```python
from build123d import *

# Parameters (mm, degrees)
SKETCH_1_R = 1


with BuildPart() as part:
    # По траектории1: sweep along a curve in space
    with BuildLine() as sweep_1_path:
        Line((0, 0, 0), (10, 0, 0))
        ThreePointArc((10, 0, 0), (12.121320344, 0, -0.878679656), (13, 0, -3))
        Line((13, 0, -3), (13, 0, -23))
        ThreePointArc((13, 0, -23), (12.121320344, 0, -25.121320344), (10, 0, -26))
        Line((10, 0, -26), (-0.116555464, 0, -26))
    # Эскиз1 → По траектории1 (sweep)
    with BuildSketch(Plane(origin=(0, 0, 0), x_dir=(0, 0, -1), z_dir=(1, 0, 0))):
        Circle(SKETCH_1_R)
    sweep(path=sweep_1_path.line)


solid = part.part
```
The listing builds one solid part. Answer for the finished solid, in the listing's coordinates (mm). A direction names the side the tool comes from. Coordinates: 2 decimals unless noted, no trailing zeros. Loops run counter-clockwise (first coordinate to the right, second up) from the corner with the lowest first, then second, coordinate; pieces in that order, holes last. Notation, with made-up numbers: (-27, 84.25) - (8, 84.25) arc R25 cw to (8, 107.25) - close; hole circle Ø9 at (20.5, 33). An arc over 180 degrees is marked (long way). Use a Markdown table: item, result. Add a question column.
1) Find the intervals of material crossed by line 1 (Z direction, x = 5.25, y = 0.15); line 2 (Z direction, x = 8.75, y = -0.45); line 3 (X direction, y = 0.6, z = -7.5), in increasing order.
2) The mould has two halves that part along Z. Classify faces 3 (the cylindrical face through (5, -1, 0)), 4 (the cylindrical face through (12, 0, -13)), 5 (the flat face through (-0.117, 0, -26)): released by +Z, released by -Z, zero draft, split by the parting line, or undercut.
3) The part is cut by section A-A, the plane y = 0.6. Give the vertices of the cut face in (x, z), and give its area (3 significant figures).
4) Given pin 1 (1 mm diameter, centred on y = 0, z = -0.5, fed in from -X), flat-ended and moving along its own axis, determine where the tip first touches the part or whether it passes through.
5) The part is cut by section C-C, the plane z = -19.75. Give the vertices of the cut face in (x, y), and give its area (3 significant figures).
6) For faces 1 (the flat face through (0, 0, 0)), 2 (the cylindrical face through (5, 0, -27)), determine the directions among +Z, -Z, +X, -X, +Y, -Y from which every point of the face is accessible in a straight line to the end or side of a thin tool.
7) The part is cut by section B-B, the plane x = 6. Give the vertices of the cut face in (y, z), and give its area (3 significant figures).
Here are the results:
| question | item | result |
|---|---|---|
| 1 | line 1 | z = -26.99 to -25.01, -0.99 to 0.99 |
| 1 | line 2 | z = -26.89 to -25.11, -0.89 to 0.89 |
| 1 | line 3 | x = 12.2 to 13.8 |
| 2 | face 3 | undercut |
| 2 | face 4 | undercut |
| 2 | face 5 | zero draft |
| 3 | outline | (-0.12, -26.8) - (10, -26.8) arc R3.8 ccw to (13.8, -23) - (13.8, -3) arc R3.8 ccw to (10, 0.8) - (0, 0.8) - (0, -0.8) - (10, -0.8) arc R2.2 cw to (12.2, -3) - (12.2, -23) arc R2.2 cw to (10, -25.2) - (-0.12, -25.2) - close |
| 3 | area | 79.3 mm^2 |
| 4 | pin 1 | stops at x = 0 |
| 5 | outline | circle Ø2 at (13, 0) |
| 5 | area | 3.14 mm^2 |
| 6 | face 1 | +Z, -X, +Y, -Y |
| 6 | face 2 | -X |
| 7 | outline | circle Ø2 at (0, -26); circle Ø2 at (0, 0) |
| 7 | area | 6.28 mm^2 |
